Could you check a few things on this drawing? It's one solid part, dimensions in mm from its lowest x, y, z. Round coordinates to 2 decimals unless told otherwise and drop trailing zeros. Loops run counter-clockwise (first coordinate to the right, second up) from the corner with the lowest first, then second, coordinate; pieces in that order, holes last. Notation, with made-up numbers: M 22.5,38 L 67.5,38 A23 ccw 67.5,46 Z; hole C -24,68.5 d8. An arc over 180 degrees is marked long. Answer as CSV lines item,"result".
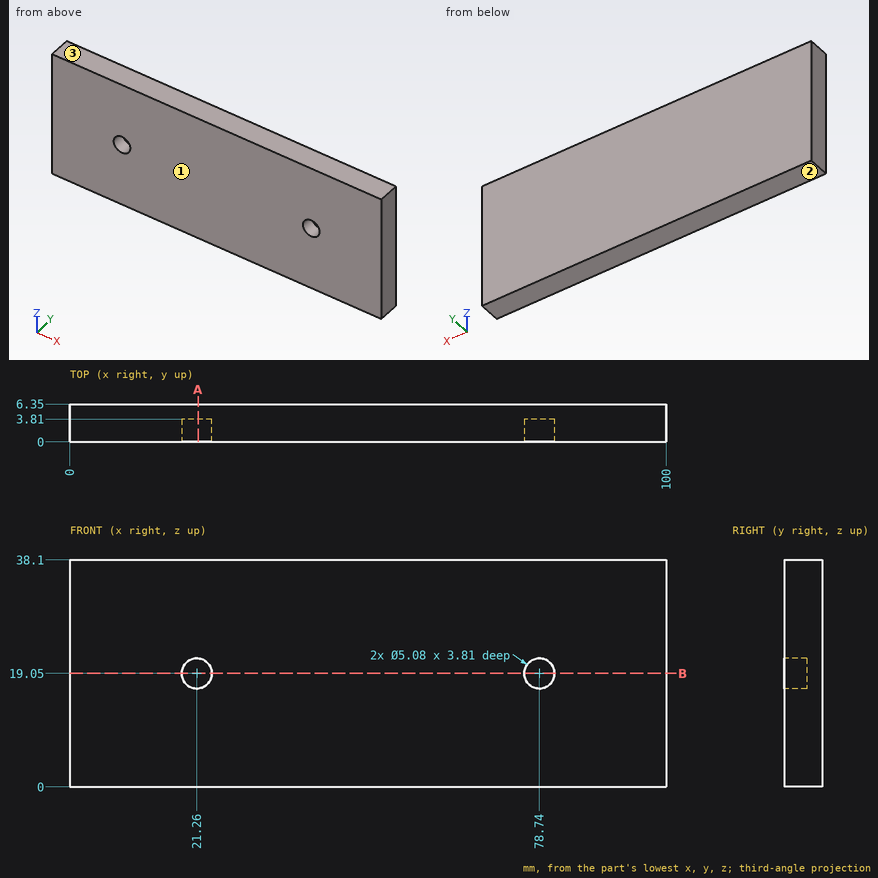
Item 1: Will this pin go through, and if not, where does the flat tip stop? pin 1 (1.5 mm diameter, centred on x = 21.5, z = 19, fed in from -Y).
Output:
pin 1,"stops at y = 3.81"
Item 2: If I drill on line 1 along X through (y, z) = (0.85, 19.05); line 2 along Z through (x, y) = (21.26, 1.3); line 3 along Y through (x, z) = (20.5, 20), over which ranges is the centre line in solid material (lowest first)? Write a range as from..to.
Output:
line 1,"x = 0..18.72, 23.8..76.2, 81.28..100"
line 2,"z = 0..16.51, 21.59..38.1"
line 3,"y = 3.81..6.35"
Item 3: If we section it at A-A on x = 21.5: Write out the boundary of the cut face in (y, z).
Output:
outline,"M 0,0 L 6.35,0 L 6.35,38.1 L 0,38.1 L 0,21.58 L 3.81,21.58 L 3.81,16.52 L 0,16.52 Z"
Item 4: We'd pull the mould along Z, two halves only. Please class the marked faces 1, 2 and 3: released by +Z, released by -Z, zero draft, split by the parting line, or undercut.
Output:
face 1,"zero draft"
face 2,"released by -Z"
face 3,"released by +Z"
Item 5: If we section it at B-B on z = 19.05: Write out the boundary of the cut face in (x, y), then the cut area to 3 significant figures.
Output:
outline,"M 0,0 L 18.72,0 L 18.72,3.81 L 23.8,3.81 L 23.8,0 L 76.2,0 L 76.2,3.81 L 81.28,3.81 L 81.28,0 L 100,0 L 100,6.35 L 0,6.35 Z"
area,"596 mm2"
